Could you check a few things on this model? Use its own coordinates, in mm. Face numbers are marked on the shaded views. A direction names the side the tool comes from. Coordinates: 2 decimals unless noted, no trailing zeros. Order: outer loops, then holes, each group sorted by start corner. A loop starts at its lowest first (then second) coordinate and runs counter-clockwise, first axis right, second up. Notation, with made-up numbers: (56.25, -7.75) - (69.25, -7.75) arc R13 cw to (69.25, -2.75) - close; hole circle Ø7 at (69.25, -28.5). An arc over 180 degrees is marked (long way). One line per item, written item: value.
from build123d import *

# Parameters (mm, degrees)
SKETCH1_W               = 58
SKETCH1_H               = 32.6
BOSS_EXTRUDE1_DEPTH     = 8
SKETCH2_W               = 20.6
SKETCH2_H               = 8
CUT_EXTRUDE1_DEPTH      = 16
SKETCH3_W               = 20.6
SKETCH3_H               = 8
CUT_EXTRUDE2_DEPTH      = 27
SKETCH5_R               = 1.6
CUT_EXTRUDE4_DEPTH      = 68.013133041
FILLET1_R               = 3
FILLET2_R               = 3
SKETCH7_W               = 15
SKETCH7_H               = 8
BOSS_EXTRUDE2_DEPTH     = 3
CUT_EXTRUDE5_DEPTH      = 3
CUT_EXTRUDE5_DEPTH_BACK = 15
SKETCH6_R               = 1.5
FILLET3_R               = 4


with BuildPart() as part:
    # Sketch1 → Boss-Extrude1 (new body)
    with BuildSketch(Plane(origin=(0, 0, 0), x_dir=(1, 0, 0), z_dir=(0, 1, 0))):
        with Locations((29, -16.3)):
            Rectangle(SKETCH1_W, SKETCH1_H)
    extrude(amount=BOSS_EXTRUDE1_DEPTH)

    # Sketch2 → Cut-Extrude1 (cut)
    with BuildSketch(Plane(origin=(58, 0, 0), x_dir=(0, 0, -1), z_dir=(1, 0, 0))):
        with Locations((-16.3, 4)):
            Rectangle(SKETCH2_W, SKETCH2_H)
    extrude(amount=-CUT_EXTRUDE1_DEPTH, mode=Mode.SUBTRACT)

    # Sketch3 → Cut-Extrude2 (cut)
    with BuildSketch(Plane.ZY):
        with Locations((16.3, 4)):
            Rectangle(SKETCH3_W, SKETCH3_H)
    extrude(amount=-CUT_EXTRUDE2_DEPTH, mode=Mode.SUBTRACT)

    # Sketch5 → Cut-Extrude4 (cut, through all)
    with BuildSketch(Plane.XY.offset(32.6)):
        with Locations((4, 4)):
            Circle(SKETCH5_R)
        with Locations((54, 4)):
            Circle(SKETCH5_R)
    extrude(amount=-CUT_EXTRUDE4_DEPTH, mode=Mode.SUBTRACT)

    # Fillet1
    fillet1_edges = [part.edges().sort_by_distance(p)[0] for p in [
        (58, 8, 29.6),
        (58, 0, 3),
        (58, 8, 3),
        (0, 0, 29.6),
        (0, 8, 29.6),
        (0, 8, 3),
        (58, 0, 29.6),
        (0, 0, 3),
    ]]
    fillet(fillet1_edges, radius=FILLET1_R)

    # Fillet2
    fillet2_edges = [part.edges().sort_by_distance(p)[0] for p in [
        (42, 4, 26.6),
        (42, 4, 6),
        (27, 4, 6),
        (27, 4, 26.6),
    ]]
    fillet(fillet2_edges, radius=FILLET2_R)

    # Sketch7 → Boss-Extrude2 (add)
    with BuildSketch(Plane.XY.offset(32.6)):
        with Locations((34.5, 4)):
            Rectangle(SKETCH7_W, SKETCH7_H)
    extrude(amount=BOSS_EXTRUDE2_DEPTH)

    # Sketch6 → Cut-Extrude5 (cut, two sides: drawn at the far end of the back side and taken through both)
    with BuildSketch(Plane.XY.offset(32.6).offset(-CUT_EXTRUDE5_DEPTH_BACK)):
        with Locations((34.5, 4)):
            Circle(SKETCH6_R)
    extrude(amount=CUT_EXTRUDE5_DEPTH + CUT_EXTRUDE5_DEPTH_BACK, mode=Mode.SUBTRACT)

    # Fillet3
    # the kernel refuses this fillet: 4 mm, written as the material it adds along each edge
    with BuildSketch(Plane(origin=(42, 8, 32.6), x_dir=(0, 0, 1), z_dir=(0, -1, 0))) as fillet3_piece_1:
        with BuildLine():
            CenterArc((4, -3.872983346), FILLET3_R, 104.477512186, 75.522487814)
            Line((0, -3.872983346), (-0.08, -3.872983346))
            Line((-0.08, -3.872983346), (-0.08, 0))
            Line((-0.08, 0), (0, 0.08))
            ThreePointArc((0, 0.08), (1.5, 0.08), (2.98, 0.077459667))
            Line((2.98, 0.077459667), (3, 0))
        make_face()
    extrude(amount=8)
    with BuildSketch(Plane(origin=(27, 0, 32.6), x_dir=(-1, 0, 0), z_dir=(0, 1, 0))) as fillet3_piece_2:
        with BuildLine():
            CenterArc((3.872983346, 4), FILLET3_R, 194.477512186, 75.522487814)
            Line((0, 3), (-0.077459667, 2.98))
            ThreePointArc((-0.077459667, 2.98), (-0.08, 1.5), (-0.08, 0))
            Line((-0.08, 0), (0, -0.08))
            Line((0, -0.08), (3.872983346, -0.08))
            Line((3.872983346, -0.08), (3.872983346, 0))
        make_face()
    extrude(amount=8)


solid = part.part
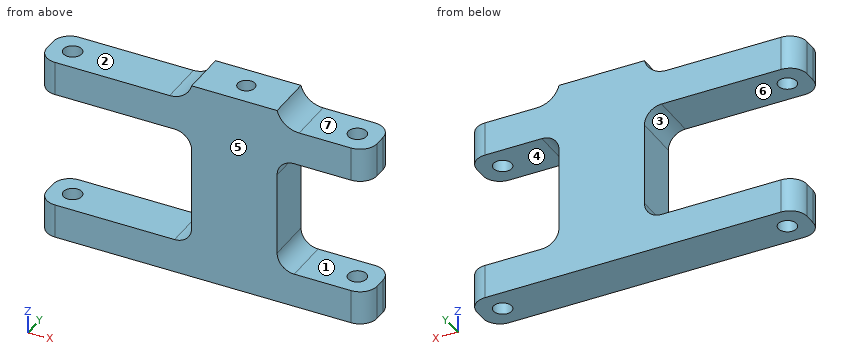
Item 1: For the marked faces 1, 2 and 3, which set-ups out of +Z, -Z, +X, -X, +Y, -Y let a thin tool reach every point of the face, with its end or its side?
Conclusion:
face 1: +X, +Y, -Y
face 2: +Z, -X, +Y, -Y
face 3: -X, +Y, -Y
Item 2: I want a section at C-C on x = 4. Please give me the cut outline in (y, z).
Conclusion:
outline: (0, 0) - (2.4, 0) - (2.4, 6) - (0, 6) - close; (0, 26.6) - (2.4, 26.6) - (2.4, 32.6) - (0, 32.6) - close; (5.6, 0) - (8, 0) - (8, 6) - (5.6, 6) - close; (5.6, 26.6) - (8, 26.6) - (8, 32.6) - (5.6, 32.6) - close
Item 3: If I drill on probe 1 along Z at (x, y) = (55.5, 2.5); probe 2 along Y at (x, z) = (34.5, 24); probe 3 along Y at (x, z) = (4, 1.75), over which ranges is the centre line in solid material (lowest first)?
Conclusion:
probe 1: 0 to 6, 26.6 to 32.6
probe 2: 0 to 2.5, 5.5 to 8
probe 3: 0 to 2.4, 5.6 to 8
Item 4: Thinking about a two-plate mould opening in Z: for the marked faces 4, 5, 6 and 7, which applies, pulls with the +Z half, pulls with the -Z half, needs draft (parallel to the pull), parting line crosses it, or undercut?
Conclusion:
face 4: undercut
face 5: needs draft
face 6: undercut
face 7: pulls with the +Z half
Item 5: I want a section at B-B on z = 32. Please give me the cut outline in (x, y), then the cut area to 3 significant figures.
Conclusion:
outline: (0, 3) arc R3 ccw to (3, 0) - (55, 0) arc R3 ccw to (58, 3) - (58, 5) arc R3 ccw to (55, 8) - (3, 8) arc R3 ccw to (0, 5) - close; hole circle Ø3.2 at (4, 4); hole circle Ø3 at (34.5, 4); hole circle Ø3.2 at (54, 4)
area: 433 mm²
Item 6: I'm going to push flat-ended pins straight in: pin 1 Ø3.5 at (x, y) = (4, 4) entering from +Z; pin 2 Ø0.9 at (x, y) = (34, 3.5) entering from +Z; pin 3 Ø4 at (y, z) = (1.5, 14) entering from +X. Where does each tip first touch, or does it pass through?
Conclusion:
pin 1: z = 32.6
pin 2: z = 17.6
pin 3: x = 42
Item 7: I want a section at A-A on x = 20. Please give me the cut outline in (y, z), then the cut area to 3 significant figures.
Conclusion:
outline: (0, 0) - (8, 0) - (8, 6) - (0, 6) - close; (0, 26.6) - (8, 26.6) - (8, 32.6) - (0, 32.6) - close
area: 96.0 mm²
Item 8: I want a section at D-D on y = 4. Give the number of separate pieces and of enclosed holes in the cut face, then the cut area to 3 significant figures.
Conclusion:
separate pieces: 5
enclosed holes: 0
area: 933 mm²
